The model under review builds one solid part; all positions refer to its coordinate system, in mm. A direction names the side the tool comes from. Coordinates: 2 decimals unless noted, no trailing zeros. Write each loop counter-clockwise with the first axis right and the second up, starting at its lowest first coordinate (ties: lowest second). Pieces come first, ordered by that corner, then holes. Notation, with made-up numbers: (37.25, 50) - (74.25, 50) arc R20 cw to (74.25, 56) - close; hole circle Ø2 at (49.25, -31.5). An arc over 180 degrees is marked (long way). Return JSON: item names as keys, results as strings. Group by question number.
(1) We need section D-D on x = 55. State the section outline as (y, z) points, then the cut area to 3 significant figures.
(2) Tool access review of faces 5 (the face through (9.36, 4.04, 5.97)), 6 (the face through (-17.54, 3.94, 8.44)): name each direction out of +Z, -Z, +X, -X, +Y, -Y from which nothing blocks a thin tool from reaching the whole face with its end or side.
(3) To check wall thickness, follow L1, parallel to X at y = 0.4, z = 0; L2, parallel to X at y = 7, z = 0; L3, parallel to X at y = 5.25, z = 7. State the ranges of each line that lie inside material, in increasing order. Write a range as from..to.
(4) We need section C-C on z = 0. State the section outline as (x, y) points.
(5) Draft analysis for pull direction X (two halves, no side actions). For faces 1 (the face through (31.077, 11.493, 1.172)), 2 (the face through (8.3, 1, -5)), 3 (the face through (21, 4, 15)), 4 (the face through (61, 4, 0)), state which applies: released by +X, released by -X, zero draft, split by the parting line, or undercut.
(6) We need section B-B on y = 4.25. State the section outline as (x, z) points.
(7) We need section A-A on x = 40. State the section outline as (y, z) points.
```python
from build123d import *

# Parameters (mm, degrees)
SKETCH1_R           = 9.5
SKETCH1_R_2         = 5
SKETCH1_R_3         = 2.6
BOSS_EXTRUDE1_DEPTH = 8
SKETCH2_R           = 11.1
CUT_EXTRUDE1_DEPTH  = 7
SKETCH3_R           = 9
SKETCH3_R_2         = 5
BOSS_EXTRUDE2_DEPTH = 4
FILLET1_R           = 3
CHAMFER1_SIZE       = 1


with BuildPart() as part:
    # Sketch1 → Boss-Extrude1 (new body)
    with BuildSketch(Plane(origin=(0, 0, 0), x_dir=(1, 0, 0), z_dir=(0, 1, 0))):
        with BuildLine():
            Line((-17, 15), (57, 15))
            ThreePointArc((57, 15), (59.828427125, 13.828427125), (61, 11))
            Line((61, 11), (61, -11))
            ThreePointArc((61, -11), (59.828427125, -13.828427125), (57, -15))
            Line((57, -15), (-17, -15))
            ThreePointArc((-17, -15), (-19.828427125, -13.828427125), (-21, -11))
            Line((-21, -11), (-21, 11))
            ThreePointArc((-21, 11), (-19.828427125, 13.828427125), (-17, 15))
        make_face()
        with Locations(Location((0, 0, 0), (0, 0, 270))):  # turned: the seam where the file's is
            Circle(SKETCH1_R, mode=Mode.SUBTRACT)
        with Locations(Location((40, 0, 0), (0, 0, 270))):  # turned: the seam where the file's is
            Circle(SKETCH1_R_2, mode=Mode.SUBTRACT)
        with Locations(Location((-15, 9, 0), (0, 0, 270))):  # turned: the seam where the file's is
            Circle(SKETCH1_R_3, mode=Mode.SUBTRACT)
        with Locations(Location((-15, -9, 0), (0, 0, 270))):  # turned: the seam where the file's is
            Circle(SKETCH1_R_3, mode=Mode.SUBTRACT)
        with Locations(Location((55, 9, 0), (0, 0, 270))):  # turned: the seam where the file's is
            Circle(SKETCH1_R_3, mode=Mode.SUBTRACT)
        with Locations(Location((55, -9, 0), (0, 0, 270))):  # turned: the seam where the file's is
            Circle(SKETCH1_R_3, mode=Mode.SUBTRACT)
    extrude(amount=BOSS_EXTRUDE1_DEPTH)

    # Sketch2 → Cut-Extrude1 (cut)
    with BuildSketch(Plane(origin=(0, 8, 0), x_dir=(1, 0, 0), z_dir=(0, 1, 0))):
        with Locations(Location((0, 0, 0), (0, 0, 270))):  # turned: the seam where the file's is
            Circle(SKETCH2_R)
    extrude(amount=-CUT_EXTRUDE1_DEPTH, mode=Mode.SUBTRACT)

    # Sketch3 → Boss-Extrude2 (add)
    with BuildSketch(Plane(origin=(0, 8, 0), x_dir=(1, 0, 0), z_dir=(0, 1, 0))):
        with Locations(Location((40, 0, 0), (0, 0, 90))):  # turned: the seam where the file's is
            Circle(SKETCH3_R)
        with Locations(Location((40, 0, 0), (0, 0, 270))):  # turned: the seam where the file's is
            Circle(SKETCH3_R_2, mode=Mode.SUBTRACT)
    extrude(amount=BOSS_EXTRUDE2_DEPTH)

    # Fillet1
    fillet1_edges = [part.edges().sort_by_distance(p)[0] for p in [
        (40, 8, 9),
    ]]
    fillet(fillet1_edges, radius=FILLET1_R)

    # Chamfer1
    chamfer1_edges = [part.edges().sort_by_distance(p)[0] for p in [
        (0, 8, -11.1),
    ]]
    chamfer(chamfer1_edges, length=CHAMFER1_SIZE)


solid = part.part
```
Ans:
{
 "1": {"outline": "(0, -15) - (8, -15) - (8, -11.6) - (0, -11.6) - close; (0, -6.4) - (8, -6.4) - (8, 6.4) - (0, 6.4) - close; (0, 11.6) - (8, 11.6) - (8, 15) - (0, 15) - close", "area": "157 mm²"},
 "2": {"face 5": "+Y", "face 6": "+Y, -Y"},
 "3": {"L1": "-21..-9.5, 9.5..35, 45..61", "L2": "-21..-11.1, 11.1..35, 45..61", "L3": "-21..-16.66, -13.34..-8.61, 8.61..53.34, 56.66..61"},
 "4": {"outline": "(-21, 0) - (-9.5, 0) - (-9.5, 1) - (-11.1, 1) - (-11.1, 7) - (-12.1, 8) - (-21, 8) - close; (9.5, 0) - (35, 0) - (35, 12) - (31, 12) - (31, 11) arc R3 cw to (28, 8) - (12.1, 8) - (11.1, 7) - (11.1, 1) - (9.5, 1) - close; (45, 0) - (61, 0) - (61, 8) - (52, 8) arc R3 cw to (49, 11) - (49, 12) - (45, 12) - close"},
 "5": {"face 1": "split by the parting line", "face 2": "undercut", "face 3": "zero draft", "face 4": "released by +X"},
 "6": {"outline": "(-21, -11) arc R4 ccw to (-17, -15) - (57, -15) arc R4 ccw to (61, -11) - (61, 11) arc R4 ccw to (57, 15) - (-17, 15) arc R4 ccw to (-21, 11) - close; hole circle Ø5.2 at (-15, -9); hole circle Ø5.2 at (-15, 9); hole circle Ø22.2 at (0, 0); hole circle Ø10 at (40, 0); hole circle Ø5.2 at (55, -9); hole circle Ø5.2 at (55, 9)"},
 "7": {"outline": "(0, -15) - (8, -15) - (8, -12) arc R3 cw to (11, -9) - (12, -9) - (12, -5) - (0, -5) - close; (0, 5) - (12, 5) - (12, 9) - (11, 9) arc R3 cw to (8, 12) - (8, 15) - (0, 15) - close"}
}
